Geometry check sheet. Reference: the model listing, model coordinates, mm. A direction names the side the tool comes from. Round coordinates to 2 decimals unless told otherwise and drop trailing zeros. Write each loop counter-clockwise with the first axis right and the second up, starting at its lowest first coordinate (ties: lowest second). Pieces come first, ordered by that corner, then holes. Notation, with made-up numbers: M 83.5,-12.5 L 135.5,-12.5 A23 ccw 135.5,3.5 Z; hole C -0.5,40 d10. An arc over 180 degrees is marked long. Answer as CSV lines item,"result". Start each with the question number.
```python
from build123d import *

# Parameters (mm, degrees)
SKETCH1_W                                  = 46
SKETCH1_H                                  = 10
BOSS_EXTRUDE1_DEPTH                        = 48
SKETCH2_W                                  = 16
SKETCH2_H                                  = 5
CUT_EXTRUDE1_DEPTH                         = 10
FILLET1_R                                  = 2
CBORE_FOR_M4_CHEESE_HEAD_SCREW1_AT_2_COUNT = 2
CBORE_FOR_M4_CHEESE_HEAD_SCREW1_AT_2_PITCH = 28
CBORE_FOR_M4_CHEESE_HEAD_SCREW1_AT_3_COUNT = 2
CBORE_FOR_M4_CHEESE_HEAD_SCREW1_AT_3_PITCH = 41.036569057
CBORE_FOR_M4_CHEESE_HEAD_SCREW1_AT_4_COUNT = 2
CBORE_FOR_M4_CHEESE_HEAD_SCREW1_AT_4_PITCH = 30
SKETCH6_R                                  = 7
CUT_EXTRUDE2_DEPTH                         = 5


with BuildPart() as part:
    # Sketch1 → Boss-Extrude1 (new body)
    with BuildSketch(Plane.XY):
        Rectangle(SKETCH1_W, SKETCH1_H)
    extrude(amount=BOSS_EXTRUDE1_DEPTH)

    # Sketch2 → Cut-Extrude1 (cut)
    with BuildSketch(Plane(origin=(0, 5, 0), x_dir=(1, 0, 0), z_dir=(0, 1, 0))):
        with Locations((0, -48)):
            Rectangle(SKETCH2_W, SKETCH2_H)
        Rectangle(SKETCH2_W, SKETCH2_H)
    extrude(amount=-CUT_EXTRUDE1_DEPTH, mode=Mode.SUBTRACT)

    # Fillet1
    fillet1_edges = [part.edges().sort_by_distance(p)[0] for p in [
        (-8, 0, 0),
        (8, 0, 0),
        (8, 0, 48),
        (-8, 0, 48),
    ]]
    fillet(fillet1_edges, radius=FILLET1_R)

    # Sketch4 → CBORE for M4 Cheese Head Screw1 (revolve, cut)
    with BuildSketch(Plane(origin=(-15, 5, 10), x_dir=(0, 0, 1), z_dir=(1, 0, 0))):
        Polygon((0, 0), (0, 11.351936393), (2.25, 10), (2.25, 2.6), (4, 2.6), (4, 0.025), (4.025, 0), align=None)
    cbore_for_m4_cheese_head_screw1 = revolve(axis=Axis((-15, 11.35, 10), (0, -1, 0)), mode=Mode.SUBTRACT)

    # CBORE for M4 Cheese Head Screw1 at 2: CBORE for M4 Cheese Head Screw1 ×2
    with Locations(*[(0, 0, i * CBORE_FOR_M4_CHEESE_HEAD_SCREW1_AT_2_PITCH) for i in range(1, CBORE_FOR_M4_CHEESE_HEAD_SCREW1_AT_2_COUNT)]):
        add(cbore_for_m4_cheese_head_screw1, mode=Mode.SUBTRACT)

    # CBORE for M4 Cheese Head Screw1 at 3: CBORE for M4 Cheese Head Screw1 ×2
    with Locations(*[Vector(0.731055268242869, 0, 0.6823182503600111) * (i * CBORE_FOR_M4_CHEESE_HEAD_SCREW1_AT_3_PITCH) for i in range(1, CBORE_FOR_M4_CHEESE_HEAD_SCREW1_AT_3_COUNT)]):
        add(cbore_for_m4_cheese_head_screw1, mode=Mode.SUBTRACT)

    # CBORE for M4 Cheese Head Screw1 at 4: CBORE for M4 Cheese Head Screw1 ×2
    with Locations(*[(i * CBORE_FOR_M4_CHEESE_HEAD_SCREW1_AT_4_PITCH, 0, 0) for i in range(1, CBORE_FOR_M4_CHEESE_HEAD_SCREW1_AT_4_COUNT)]):
        add(cbore_for_m4_cheese_head_screw1, mode=Mode.SUBTRACT)

    # Sketch6 → Cut-Extrude2 (cut)
    with BuildSketch(Plane(origin=(0, 5, 0), x_dir=(1, 0, 0), z_dir=(0, 1, 0))):
        with Locations(Location((0, -24, 0), (0, 0, 270))):
            Circle(SKETCH6_R)
    extrude(amount=-CUT_EXTRUDE2_DEPTH, mode=Mode.SUBTRACT)


solid = part.part
```
1) Section check D-D, the plane z = 24. Record the cut outline in (x, y).
2) Mould release check, pull along X, two halves, no side actions. Record for faces 1 (the flat face through (23, 0, 24)), 2 (the flat face through (0, 0, 45.5)), 3 (the flat face through (-17, 0, 48)), 4 (the cylindrical face through (-8.6, 0.07, 0.57)): released by +X, released by -X, zero draft, split by the parting line, or undercut.
3) Section check B-B, the plane z = 10. Record the cut outline in (x, y) (3 decimals), plus the area to 3 significant figures.
4) Scan lines: line 1 (Z direction, x = 15, y = 0.5); line 2 (Z direction, x = -15, y = 3.8); line 3 (X direction, y = -0.75, z = 38). Record each from-to range of solid material in increasing order. Write a range as from..to.
5) Go/stop test with flat-tipped pins: pin 1 (3 mm diameter, centred on x = -2.5, y = -2.5, fed in from +Z); pin 2 (1.5 mm diameter, centred on x = -7.5, y = -3.5, fed in from -Z); pin 3 (2.5 mm diameter, centred on x = -14.5, z = 10.5, fed in from +Y); pin 4 (7 mm diameter, centred on x = -15, z = 10, fed in from +Y). Record where each tip stops, or that it passes through.
6) Section check C-C, the plane y = 1. Record the cut outline in (x, z), plus the area to 3 significant figures.
7) Access from +Z, -Z, +X, -X, +Y, -Y to the whole of each face (thin tool, end or side, straight path). Record for faces 5 (the flat face through (0, 0, 2.5)), 6 (the flat face through (-13, 2.4, 8)), 7 (the cylindrical face through (8.6, 0.07, 47.43)).
8) Section check A-A, the plane x = 15. Record the cut outline in (y, z) (3 decimals), plus the area to 3 significant figures.
Results:
1,outline,"M -23,-5 L 23,-5 L 23,5 L 7,5 L 7,0 L -7,0 L -7,5 L -23,5 Z"
2,face 1,"released by +X"
2,face 2,"undercut"
2,face 3,"zero draft"
2,face 4,"undercut"
3,outline,"M -23,-5 L -17.25,-5 L -17.25,2.4 L -19,2.4 L -19,4.975 L -19.025,5 L -23,5 Z; M -12.75,-5 L 12.75,-5 L 12.75,2.4 L 11,2.4 L 11,4.975 L 10.975,5 L -10.975,5 L -11,4.975 L -11,2.4 L -12.75,2.4 Z; M 17.25,-5 L 23,-5 L 23,5 L 19.025,5 L 19,4.975 L 19,2.4 L 17.25,2.4 Z"
3,area,"352 mm^2"
4,line 1,"z = 0..7.75, 12.25..35.75, 40.25..48"
4,line 2,"z = 0..6, 14..34, 42..48"
4,line 3,"x = -23..-17.25, -12.75..12.75, 17.25..23"
5,pin 1,"stops at z = 45.5"
5,pin 2,"stops at z = 1.03"
5,pin 3,"passes through"
5,pin 4,"stops at y = 2.4"
6,outline,"M -23,0 L -10,0 A2 ccw -8,2 L -8,2.5 L 8,2.5 L 8,2 A2 ccw 10,0 L 23,0 L 23,48 L 10,48 A2 ccw 8,46 L 8,45.5 L -8,45.5 L -8,46 A2 ccw -10,48 L -23,48 Z; hole C -15,10 d4.5; hole C -15,38 d4.5; hole C 0,24 d14; hole C 15,10 d4.5; hole C 15,38 d4.5"
6,area,"1,910 mm^2"
7,face 5,"-Z, +Y, -Y"
7,face 6,"+Y"
7,face 7,"+Z, +Y, -Y"
8,outline,"M -5,0 L 5,0 L 5,5.975 L 4.975,6 L 2.4,6 L 2.4,7.75 L -5,7.75 Z; M -5,12.25 L 2.4,12.25 L 2.4,14 L 4.975,14 L 5,14.025 L 5,33.975 L 4.975,34 L 2.4,34 L 2.4,35.75 L -5,35.75 Z; M -5,40.25 L 2.4,40.25 L 2.4,42 L 4.975,42 L 5,42.025 L 5,48 L -5,48 Z"
8,area,"372 mm^2"
